from build123d import *

# Parameters (mm, degrees)
SKETCH_1_W          = 40
SKETCH_1_H          = 20
EXTRUDE_1_DEPTH     = 26
EXTRUDE_2_DEPTH     = 2.5
SKETCH_3_W          = 40
SKETCH_3_H          = 20
EXTRUDE_3_DEPTH     = 7.5
EXTRUDE_4_DEPTH     = 1.3
SKETCH_5_R          = 9.5
EXTRUDE_5_DEPTH     = 1.5
SKETCH_6_R          = 3
EXTRUDE_6_DEPTH     = 4.2
SKETCH_7_W          = 8
SKETCH_7_H          = 3
EXTRUDE_7_DEPTH     = 1
SKETCH_8_W          = 7.6
SKETCH_8_H          = 2.6
EXTRUDE_8_DEPTH     = 3
SKETCH_9_R          = 0.75
EXTRUDE_9_DEPTH     = 5
SKETCH_10_R         = 1.5
CUT_EXTRUDE_1_DEPTH = 3


with BuildPart() as part:
    # 스케치1 → 보스-돌출1 (new body)
    with BuildSketch(Plane(origin=(0, 0, 0), x_dir=(1, 0, 0), z_dir=(0, 1, 0))):
        Rectangle(SKETCH_1_W, SKETCH_1_H)
    extrude(amount=EXTRUDE_1_DEPTH)

    # 스케치2 → 보스-돌출2 (add)
    with BuildSketch(Plane(origin=(0, 26, 0), x_dir=(1, 0, 0), z_dir=(0, 1, 0))):
        with BuildLine():
            Line((-27, 10), (27, 10))
            Line((27, 10), (27, 6.25))
            Line((27, 6.25), (25.868643032, 6.25))
            ThreePointArc((25.868643032, 6.25), (21.751817004, 5), (25.868643032, 3.75))
            Line((25.868643032, 3.75), (27, 3.75))
            Line((27, 3.75), (27, -3.75))
            Line((27, -3.75), (25.866173833, -3.75))
            ThreePointArc((25.866173833, -3.75), (21.753868932, -5), (25.866173833, -6.25))
            Line((25.866173833, -6.25), (27, -6.25))
            Line((27, -6.25), (27, -10))
            Line((27, -10), (-27, -10))
            Line((-27, -10), (-27, -6.25))
            Line((-27, -6.25), (-25.870828693, -6.25))
            ThreePointArc((-25.870828693, -6.25), (-21.75, -5), (-25.870828693, -3.75))
            Line((-25.870828693, -3.75), (-27, -3.75))
            Line((-27, -3.75), (-27, 3.75))
            Line((-27, 3.75), (-25.870828693, 3.75))
            ThreePointArc((-25.870828693, 3.75), (-21.75, 5), (-25.870828693, 6.25))
            Line((-25.870828693, 6.25), (-27, 6.25))
            Line((-27, 6.25), (-27, 10))
        make_face()
    extrude(amount=EXTRUDE_2_DEPTH)

    # 스케치3 → 보스-돌출3 (add)
    with BuildSketch(Plane(origin=(0, 28.5, 0), x_dir=(1, 0, 0), z_dir=(0, 1, 0))):
        Rectangle(SKETCH_3_W, SKETCH_3_H)
    extrude(amount=EXTRUDE_3_DEPTH)

    # 스케치4 → 보스-돌출4 (add)
    with BuildSketch(Plane(origin=(0, 36, 0), x_dir=(1, 0, 0), z_dir=(0, 1, 0))):
        with BuildLine():
            Line((-11.105930899, 7.466746492), (9.486550883, 9.4559828))
            ThreePointArc((9.486550883, 9.4559828), (19.9, -1.9624e-05), (9.486511816, -9.455979026))
            Line((9.486511816, -9.455979026), (-11.105960469, -7.466657767))
            ThreePointArc((-11.105960469, -7.466657767), (-17.9, 5.7816e-05), (-11.105930899, 7.466746492))
        make_face()
    extrude(amount=EXTRUDE_4_DEPTH)

    # 스케치5 → 보스-돌출5 (add)
    with BuildSketch(Plane(origin=(0, 37.3, 0), x_dir=(1, 0, 0), z_dir=(0, 1, 0))):
        with Locations(Location((10.4, 0, 0), (0, 0, 95.517659112))):
            Circle(SKETCH_5_R)
    extrude(amount=EXTRUDE_5_DEPTH)

    # 스케치6 → 보스-돌출6 (add)
    with BuildSketch(Plane(origin=(0, 38.8, 0), x_dir=(1, 0, 0), z_dir=(0, 1, 0))):
        with Locations(Location((10.4, 0, 0), (0, 0, 270))):
            Circle(SKETCH_6_R)
    extrude(amount=EXTRUDE_6_DEPTH)

    # 스케치7 → 보스-돌출7 (add)
    with BuildSketch(Plane(origin=(20, 0, 0), x_dir=(0, 0, -1), z_dir=(1, 0, 0))):
        with Locations((0, 3.5)):
            Rectangle(SKETCH_7_W, SKETCH_7_H)
    extrude(amount=EXTRUDE_7_DEPTH)

    # 스케치8 → 보스-돌출8 (add)
    with BuildSketch(Plane(origin=(21, 0, 0), x_dir=(0, 0, -1), z_dir=(1, 0, 0))):
        with Locations((0, 3.5)):
            Rectangle(SKETCH_8_W, SKETCH_8_H)
    extrude(amount=EXTRUDE_8_DEPTH)

    # 스케치9 → 보스-돌출9 (add)
    with BuildSketch(Plane(origin=(24, 0, 0), x_dir=(0, 0, -1), z_dir=(1, 0, 0))):
        with Locations((0, 3.505070748)):
            Circle(SKETCH_9_R)
        with Locations((-1.999991967, 3.499402084)):
            Circle(SKETCH_9_R)
        with Locations((1.99999474, 3.500483844)):
            Circle(SKETCH_9_R)
    extrude(amount=EXTRUDE_9_DEPTH)

    # 스케치10 → 컷-돌출1 (cut)
    with BuildSketch(Plane(origin=(0, 43, 0), x_dir=(1, 0, 0), z_dir=(0, 1, 0))):
        with Locations(Location((10.4, 0, 0), (0, 0, 270))):
            Circle(SKETCH_10_R)
    extrude(amount=-CUT_EXTRUDE_1_DEPTH, mode=Mode.SUBTRACT)


solid = part.part
Design review of the part built by this model. Coordinates are the model's own, in mm. A direction names the side the tool comes from. Coordinates: 2 decimals unless noted, no trailing zeros. Order: outer loops, then holes, each group sorted by start corner. A loop starts at its lowest first (then second) coordinate and runs counter-clockwise, first axis right, second up. Notation, with made-up numbers: (-7, -32) - (-2, -32) arc R30 cw to (-2, 2) - close; hole circle Ø5 at (45.5, 11.25). An arc over 180 degrees is marked (long way). Put each result on its own line as item: value.
1) Take a section at D-D, the plane y = 13. Give the boundary of the cut face in (x, z), and give its area (3 significant figures).
Response values:
outline: (-20, -10) - (20, -10) - (20, 10) - (-20, 10) - close
area: 800 mm²
2) Wall thickness on L1, parallel to Z at x = 24, y = 27; L2, parallel to X at y = 27.7, z = 5; L3, parallel to X at y = 21.5, z = -8: over which ranges is each line inside the solid? List them lowest first. Write a range as from..to.
Response values:
L1: z = -10..-7.25, -2.75..2.75, 7.25..10
L2: x = -21.75..21.75
L3: x = -20..20
3) Take a section at B-B, the plane x = 10.4. Give the boundary of the cut face in (y, z), and give its area (3 significant figures).
Response values:
outline: (0, -10) - (36, -10) - (36, -9.5) - (38.8, -9.5) - (38.8, -3) - (43, -3) - (43, -1.5) - (40, -1.5) - (40, 1.5) - (43, 1.5) - (43, 3) - (38.8, 3) - (38.8, 9.5) - (36, 9.5) - (36, 10) - (0, 10) - close
area: 789 mm²
4) Take a section at A-A, the plane x = -24. Give the boundary of the cut face in (y, z), and give its area (3 significant figures).
Response values:
outline: (26, -10) - (28.5, -10) - (28.5, -7.25) - (26, -7.25) - close; (26, -2.75) - (28.5, -2.75) - (28.5, 2.75) - (26, 2.75) - close; (26, 7.25) - (28.5, 7.25) - (28.5, 10) - (26, 10) - close
area: 27.5 mm²
5) Tool access review of faces 1 (the face through (-6, 36, 9)), 2 (the face through (26.4, 27.2, 6.25)), 3 (the face through (-23, 26, 0)), 4 (the face through (20, 32, 0)), 5 (the face through (-26.4, 27.2, 6.25)): name each direction out of +Z, -Z, +X, -X, +Y, -Y from which nothing blocks a thin tool from reaching the whole face with its end or side.
Response values:
face 1: +Y
face 2: +X, +Y, -Y
face 3: +Z, -Z, -X, -Y
face 4: +Z, -Z, +X, +Y
face 5: -X, +Y, -Y
6) Insertion check: P1, Ø10, axis at x = -3.5, z = -5, coming from the +Y side; P2, Ø6, axis at y = 15.5, z = 1.5, coming from the -X side; P3, Ø3, axis at y = 27, z = 7.5, coming from the +X side. Each pin has a flat end and moves straight along its axis. Give the tip position at first contact, or say it passes through.
Response values:
P1: stops at y = 37.3
P2: stops at x = -20
P3: stops at x = 27
7) Take a section at C-C, the plane z = 8.75. Give the boundary of the cut face in (x, y), and give its area (3 significant figures).
Response values:
outline: (-27, 26) - (-20, 26) - (-20, 0) - (20, 0) - (20, 26) - (27, 26) - (27, 28.5) - (20, 28.5) - (20, 36) - (14.1, 36) - (14.1, 38.8) - (6.7, 38.8) - (6.7, 37.3) - (2.18, 37.3) - (2.18, 36) - (-20, 36) - (-20, 28.5) - (-27, 28.5) - close
area: 1,500 mm²
